```python
from build123d import *

# Parameters (mm, degrees)
F0_W     = 37.5
F0_H     = 17
F1_DEPTH = 3


# Not quite as in the source:
# - a feature names something its author has since deleted; it is built from what else it names


with BuildPart() as f1:
    # F0 (on Top) → F1 (new body)
    with BuildSketch(Plane.XY):
        with Locations((18.75, 45.5)):
            Rectangle(F0_W, F0_H)
        Polygon((95, 37), (37.5, 37), (37.5, 0), (40, 4.5), (47.5, 4.5), (55, 4.5), (57.5, 0), (95, 0), (95, 17), (91, 19.5), (91, 27), (91, 34.5), align=None)
        Polygon((40, 49.5), (37.5, 54), (37.5, 37), (95, 37), (95, 54), (57.5, 54), (55, 49.5), (47.5, 49.5), align=None)
        Polygon((37.5, 37), (0, 37), (4, 34.5), (4, 27), (4, 19.5), (0, 17), (0, 0), (37.5, 0), align=None)
    extrude(amount=F1_DEPTH)


solid = f1.part
```
Build history of the part. All positions in model axes, mm. A direction names the side the tool comes from. Give positions to 0.01 mm unless a question says otherwise; leave off trailing zeros. Order: outer loops, then holes, each group sorted by start corner. A loop starts at its lowest first (then second) coordinate and runs counter-clockwise, first axis right, second up. Notation, with made-up numbers: M -6,-1.75 L 14,-1.75 A6 ccw 14,4.25 Z; hole C 77.5,-40 d7. An arc over 180 degrees is marked long. Write item = value, one per line. Start each with the question number.
(1) Slice it at A-A on z = 1.6. Write the cut outline in (x, y), plus the area to 3 significant figures.
(2) Pin check, flat tips, straight feed: pin 1 Ø0.9 at (x, z) = (50.5, 1) entering from -Y; pin 2 Ø0.9 at (x, z) = (46, 2) entering from +Y; pin 3 Ø1.5 at (y, z) = (28.5, 1) entering from +X. Stop position of each tip, or through.
(3) Slice it at B-B on y = 32. Write the cut outline in (x, z), plus the area to 3 significant figures.
(4) Which spindle directions (+Z, -Z, +X, -X, +Y, -Y) get a long thin tool onto all of the face, cutting with end or side? Do faces 4 (the flat face through (2.03, 18.27, 1.48)), 5 (the flat face through (92.97, 35.73, 1.48)), 6 (the flat face through (38.768, 51.718, 1.479)). Say none if no direction does.
(5) Probe L1, parallel to Y at x = 54.5, z = 1.4; L2, parallel to X at y = 30, z = 2.6; L3, parallel to X at y = 51, z = 1. List the from-to ranges inside material, lowest first. Write a range as [from, to].
(6) Two-plate mould, pull along Y, no slides. Class faces 1 (the flat face through (4, 27, 1)), 2 (the flat face through (56.268, 51.782, 1.479)), 3 (the flat face through (47, 4.5, 1)): released by +Y, released by -Y, zero draft, split by the parting line, or undercut.
Responses:
q1.outline = M 0,0 L 37.5,0 L 40,4.5 L 55,4.5 L 57.5,0 L 95,0 L 95,17 L 91,19.5 L 91,34.5 L 95,37 L 95,54 L 57.5,54 L 55,49.5 L 40,49.5 L 37.5,54 L 0,54 L 0,37 L 4,34.5 L 4,19.5 L 0,17 Z
q1.area = 4,830 mm2
q2.pin_1 = 4.5
q2.pin_2 = 49.5
q2.pin_3 = 91
q3.outline = M 4,0 L 91,0 L 91,3 L 4,3 Z
q3.area = 261 mm2
q4.face_4 = +Z, -Z, -X
q4.face_5 = +Z, -Z, +X
q4.face_6 = +Z, -Z, +Y
q5.L1 = [4.5, 49.5]
q5.L2 = [4, 91]
q5.L3 = [0, 39.17], [55.83, 95]
q6.face_1 = undercut
q6.face_2 = released by +Y
q6.face_3 = released by -Y
